from build123d import *

# Parameters (mm, degrees)
SKETCH_1_R          = 5.5
EXTRUDE_1_DEPTH     = 2.2
SKETCH_2_R          = 3
EXTRUDE_3_DEPTH     = 12
CHAMFER_2_SIZE      = 0.2
CHAMFER_3_SIZE      = 1.9
CUT_EXTRUDE_2_DEPTH = 3


with BuildPart() as part:
    # 草图1 → 凸台-拉伸1 (new body)
    with BuildSketch(Plane(origin=(0, 0, 0), x_dir=(0, 0, -1), z_dir=(1, 0, 0))):
        Circle(SKETCH_1_R)
    extrude(amount=EXTRUDE_1_DEPTH)

    # 草图2 → 凸台-拉伸3 (add)
    with BuildSketch(Plane.ZY):
        Circle(SKETCH_2_R)
    extrude(amount=EXTRUDE_3_DEPTH)

    # 倒角2
    chamfer_2_edges = [part.edges().sort_by_distance(p)[0] for p in [
        (-12, 0, -3),
    ]]
    chamfer(chamfer_2_edges, length=CHAMFER_2_SIZE)

    # 倒角3
    chamfer_3_edges = [part.edges().sort_by_distance(p)[0] for p in [
        (0, 0, 5.5),
    ]]
    chamfer(chamfer_3_edges, length=CHAMFER_3_SIZE)

    # 草图5 → 切除-拉伸2 (cut)
    with BuildSketch(Plane(origin=(2.2, 0, 0), x_dir=(0, 0, -1), z_dir=(1, 0, 0))):
        Polygon((0.3, 0.3), (1.9, 0.3), (1.9, -0.3), (0.3, -0.3), (0.3, -1.9), (-0.3, -1.9), (-0.3, -0.3), (-1.9, -0.3), (-1.9, 0.3), (-0.3, 0.3), (-0.3, 1.9), (0.3, 1.9), align=None)
    extrude(amount=-CUT_EXTRUDE_2_DEPTH, mode=Mode.SUBTRACT)


solid = part.part
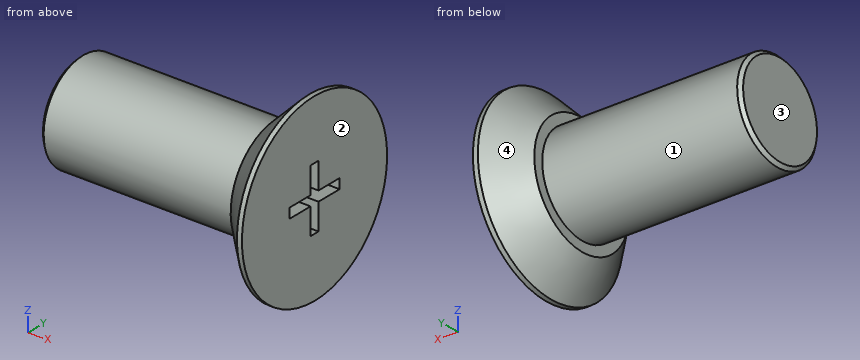
Work out the finished part from the listing and answer in its coordinate system (mm). Face numbers are marked on the shaded views. A direction names the side the tool comes from. Round coordinates to 2 decimals unless told otherwise and drop trailing zeros. Write each loop counter-clockwise with the first axis right and the second up, starting at its lowest first coordinate (ties: lowest second). Pieces come first, ordered by that corner, then holes. Notation, with made-up numbers: (14, 45) - (42, 45) arc R17 ccw to (42, 72) - close; hole circle Ø4 at (39, 25). An arc over 180 degrees is marked (long way). Answer in a Markdown table with one row per item. Add a question column.
1. A cutting plane is placed at C-C, the plane x = -2.25. Determine the outline of the cut face in (y, z).
2. The mould has two halves that part along Y. Classify the marked faces 3 and 4: +Y half, -Y half, draft (parallel to the pull), parting line (faces both ways), or undercut.
3. A cutting plane is placed at A-A, the plane y = 0. Determine the outline of the cut face in (x, z).
4. For the marked faces 1 and 2, determine the directions among +Z, -Z, +X, -X, +Y, -Y from which every point of the face is accessible in a straight line to the end or side of a thin tool.
5. Find the intervals of material crossed by line 1 along Y through (x, z) = (0.5, -1.75); line 2 along Y through (x, z) = (-7.5, 0); line 3 along X through (y, z) = (2.5, 2), in increasing order. Write a range as from..to.
6. Given pin 1 (2 mm diameter, centred on x = -5, z = -2.5, fed in from -Y); pin 2 (1.8 mm diameter, centred on x = 0.5, y = 1, fed in from +Z); pin 3 (2 mm diameter, centred on y = 0, z = 1, fed in from +X); pin 4 (1.8 mm diameter, centred on x = 0.5, z = 1, fed in from +Y), each flat-ended and moving along its own axis, determine where each tip first touches the part or whether it passes through.
Worked out:
| question | item | result |
|---|---|---|
| 1 | outline | circle Ø6 at (0, 0) |
| 2 | face 3 | draft |
| 2 | face 4 | parting line |
| 3 | outline | (-12, -2.8) - (-11.8, -3) - (0, -3) - (0, -3.6) - (1.9, -5.5) - (2.2, -5.5) - (2.2, -1.9) - (-0.8, -1.9) - (-0.8, 1.9) - (2.2, 1.9) - (2.2, 5.5) - (1.9, 5.5) - (0, 3.6) - (0, 3) - (-11.8, 3) - (-12, 2.8) - close |
| 4 | face 1 | -X |
| 4 | face 2 | +Z, -Z, +X, +Y, -Y |
| 5 | line 1 | -3.71..-0.3, 0.3..3.71 |
| 5 | line 2 | -3..3 |
| 5 | line 3 | 0..2.2 |
| 6 | pin 1 | y = -2.6 |
| 6 | pin 2 | z = 4.91 |
| 6 | pin 3 | x = 2.2 |
| 6 | pin 4 | y = 4.91 |
